Design review of the part built by this model. Coordinates are the model's own, in mm. A direction names the side the tool comes from. Give positions to 0.01 mm unless a question says otherwise; leave off trailing zeros. Loops run counter-clockwise (first coordinate to the right, second up) from the corner with the lowest first, then second, coordinate; pieces in that order, holes last.
from build123d import *

# Parameters (mm, degrees)
SKETCH_2_W              = 244
SKETCH_2_H              = 25
SM_BASE_FLANGE_1_DEPTH  = 1.5
SM_EDGE_FLANGE_1_DEPTH  = 26
HOLE_WIZARD_5_2_5_2_1_D = 5.2
HOLE_WIZARD_M3_1_D      = 2.5
FILLET_1_R              = 3


# Sheet-metal steps are written as plain solids
with BuildPart() as part:
    # Sketch 2 → 基体-法兰1 (new body)
    with BuildSketch(Plane(origin=(0, 0, 0), x_dir=(1, 0, 0), z_dir=(0, 1, 0))):
        Rectangle(SKETCH_2_W, SKETCH_2_H)
    extrude(amount=-SM_BASE_FLANGE_1_DEPTH)

    # 边线-法兰1 section (across the edge) → 边线-法兰1 (add)
    with BuildSketch(Plane(origin=(-13, 0, 20.5), x_dir=(0, 0, -1), z_dir=(1, 0, 0))):
        with BuildLine():
            Line((0, 1), (0, 58.5))
            Line((0, 58.5), (1.5, 58.5))
            Line((1.5, 58.5), (1.5, 1))
            ThreePointArc((1.5, 1), (1.792893219, 0.292893219), (2.5, 0))
            Line((2.5, 0), (8, 0))
            Line((8, 0), (8, -1.5))
            Line((8, -1.5), (2.5, -1.5))
            ThreePointArc((2.5, -1.5), (0.732233047, -0.767766953), (0, 1))
        make_face()
    extrude(amount=SM_EDGE_FLANGE_1_DEPTH)

    # Ø5.2 (5.2) 直径孔1 (through all)
    with Locations(Plane(origin=(0, -1.5, 0), x_dir=(-1, 0, 0), z_dir=(0, -1, 0))):
        with Locations((116, -5), (-116, -5)):
            Hole(HOLE_WIZARD_5_2_5_2_1_D / 2)

    # M3 螺纹孔1 (through all)
    with Locations(Plane.XY.offset(20.5)):
        with Locations((-9.25, 27), (9.25, 27)):
            Hole(HOLE_WIZARD_M3_1_D / 2)

    # 圆角1
    fillet_1_edges = [part.edges().sort_by_distance(p)[0] for p in [
        (122, -0.75, -12.5),
        (122, -0.75, 12.5),
        (13, 58.5, 19.75),
        (-13, 58.5, 19.75),
        (-122, -0.75, 12.5),
        (-122, -0.75, -12.5),
    ]]
    fillet(fillet_1_edges, radius=FILLET_1_R)


solid = part.part
Q1. Wall thickness on line 1 (Z direction, x = -116, y = -0.3); line 2 (Z direction, x = -9.5, y = 2.5); line 3 (Y direction, x = 27, z = -7): over which ranges is each line inside the solid? List them lowest first.
Results:
line 1: z = -12.5 to 2.4, 7.6 to 12.5
line 2: z = 19 to 20.5
line 3: y = -1.5 to 0
Q2. Take a section at C-C (x = -95.5). Give the boundary of the cut face in (y, z).
Results:
outline: (-1.5, -12.5) - (0, -12.5) - (0, 12.5) - (-1.5, 12.5) - close
Q3. Draft analysis for pull direction Z (two halves, no side actions). For faces 4 (the face through (0, 29, 20.5)), 5 (the face through (13, 22.9, 19.4)), 6 (the face through (118.48, -0.74, 4.22)), 7 (the face through (0, 30, 19)), state which applies: pulls with the +Z half, pulls with the -Z half, needs draft (parallel to the pull), parting line crosses it, or undercut.
Results:
face 4: pulls with the +Z half
face 5: needs draft
face 6: undercut
face 7: pulls with the -Z half
Q4. Take a section at A-A (x = 116). Give the boundary of the cut face in (y, z), plus the area to 3 significant figures.
Results:
outline: (-1.5, -12.5) - (0, -12.5) - (0, 2.4) - (-1.5, 2.4) - close; (-1.5, 7.6) - (0, 7.6) - (0, 12.5) - (-1.5, 12.5) - close
area: 29.7 mm2
Q5. Insertion check: pin 1 (7 mm diameter, centred on x = 116, z = 5, fed in from +Y); pin 2 (3 mm diameter, centred on x = -9.25, y = 27, fed in from -Z); pin 3 (1.6 mm diameter, centred on x = -45, y = -0.5, fed in from +Z). Each pin has a flat end and moves straight along its axis. Give the tip position at first contact, or say it passes through.
Results:
pin 1: stops at y = 0
pin 2: stops at z = 19
pin 3: stops at z = 12.5
Q6. Tool access review of faces 1 (the face through (-2, 0, -1)), 2 (the face through (-13, 22.9, 19.4)), 3 (the face through (-113.52, -0.74, 4.22)): name each direction out of +Z, -Z, +X, -X, +Y, -Y from which nothing blocks a thin tool from reaching the whole face with its end or side.
Results:
face 1: -Z, +X, -X, +Y
face 2: +Z, -X, +Y, -Y
face 3: +Y, -Y
Q7. Take a section at B-B (y = 31). Give the boundary of the cut face in (x, z).
Results:
outline: (-13, 19) - (13, 19) - (13, 20.5) - (-13, 20.5) - close
